Design review of the part built by this model. Coordinates are the model's own, in mm. A direction names the side the tool comes from. Round coordinates to 2 decimals unless told otherwise and drop trailing zeros. Loops run counter-clockwise (first coordinate to the right, second up) from the corner with the lowest first, then second, coordinate; pieces in that order, holes last. Notation, with made-up numbers: (-16.5, 82) - (-5.5, 82) arc R16 cw to (-5.5, 104) - close; hole circle Ø6 at (29, 39). An arc over 180 degrees is marked (long way). Answer as CSV lines item,"result". Start each with the question number.
(1) Consider section D-D (y = 2.5). Give the boundary of the cut face in (x, z).
(2) Consider section A-A (z = 0). Give the boundary of the cut face in (x, y) (3 decimals).
(3) Mouldability with a two-part tool opening along X and no side actions: class faces 1 (the cylindrical face through (7.7, 22.9, 10.1)), 2 (the flat face through (-3, 25.4, -3)), 3 (the flat face through (-1, 3.505, -1)) as released by +X, released by -X, zero draft, split by the parting line, or undercut.
(4) Consider section C-C (z = 9). Give the boundary of the cut face in (x, y), and give its area (3 significant figures).
(5) Consider section B-B (x = 0). Give the boundary of the cut face in (y, z) (3 decimals), and give its area (3 significant figures).
(6) For P1, Ø3, axis at x = -2.5, y = 23, coming from the -Z side; P2, Ø4, axis at y = 9, z = -3, coming from the +X side; P3, Ø4, axis at x = 0, z = 9.525, coming from the -Y side; P4, Ø8, axis at x = 0, z = 0, coming from the +Y side, all flat-tipped, find the tip position at first contact; note any pin that passes through.
(7) For faces 4 (the cylindrical face through (-3.778, 14.84, 0.496)), 5 (the cylindrical face through (3.86, 10.3, 5.04)), 6 (the cylindrical face through (0.773, 22.896, 10.533)), list the 3-axis set-ups (+Z, -Z, +X, -X, +Y, -Y) from which the entire face can be reached by the end or side of a thin tool; tool diameter is ignored.
(8) Wall thickness on L1, parallel to X at y = 23.75, z = 1; L2, parallel to Y at x = -9.75, z = 5.25; L3, parallel to Z at x = 6.5, y = 24.5: over which ranges is each line inside the solid? List them lowest first.
from build123d import *

# Parameters (mm, degrees)
SKETCH2_R          = 2.54
CUT_EXTRUDE1_DEPTH = 3.5052
SKETCH4_R          = 1.27
CUT_EXTRUDE2_DEPTH = 32.108519733
CIRPATTERN1_COUNT  = 8


with BuildPart() as part:
    # Sketch1 → Revolve1 (revolve)
    with BuildSketch(Plane.XY, mode=Mode.PRIVATE) as revolve1_sk:
        Polygon((3.81, 25.4), (3.81, 4.572), (0.635, 4.572), (0.635, 0), (6.35, 0), (6.35, 20.32), (12.7, 20.32), (12.7, 25.4), align=None)
    revolve(revolve1_sk.sketch.rotate(Axis((0, 0, 0), (0, 1, 0)), 90), axis=Axis((0, 0, 0), (0, 1, 0)))

    # Sketch2 → Cut-Extrude1 (cut)
    with BuildSketch(Plane.XZ):
        with Locations(Location((0, 0, 0), (0, 0, 270))):
            Circle(SKETCH2_R)
    extrude(amount=-CUT_EXTRUDE1_DEPTH, mode=Mode.SUBTRACT)

    # Sketch4 → Cut-Extrude2 (cut, through all)
    with BuildSketch(Plane(origin=(0, 25.4, 0), x_dir=(1, 0, 0), z_dir=(0, 1, 0))):
        with Locations(Location((0, 9.525, 0), (0, 0, 270))):
            Circle(SKETCH4_R)
    cut_extrude2 = extrude(amount=-CUT_EXTRUDE2_DEPTH, mode=Mode.SUBTRACT)

    # CirPattern1: Cut-Extrude2 ×8 about axis
    cirpattern1_axis = Axis((0, 0, 0), (0, 1, 0))
    for i in range(1, CIRPATTERN1_COUNT):
        add(cut_extrude2.rotate(cirpattern1_axis, i * 360 / CIRPATTERN1_COUNT), mode=Mode.SUBTRACT)


solid = part.part
Determined:
1,outline,"circle Ø12.7 at (0, 0); hole circle Ø5.08 at (0, 0)"
2,outline,"(-12.7, 20.32) - (-10.795, 20.32) - (-10.795, 25.4) - (-12.7, 25.4) - close; (-8.255, 20.32) - (-6.35, 20.32) - (-6.35, 0) - (-2.54, 0) - (-2.54, 3.505) - (-0.635, 3.505) - (-0.635, 4.572) - (-3.81, 4.572) - (-3.81, 25.4) - (-8.255, 25.4) - close; (0.635, 3.505) - (2.54, 3.505) - (2.54, 0) - (6.35, 0) - (6.35, 20.32) - (8.255, 20.32) - (8.255, 25.4) - (3.81, 25.4) - (3.81, 4.572) - (0.635, 4.572) - close; (10.795, 20.32) - (12.7, 20.32) - (12.7, 25.4) - (10.795, 25.4) - close"
3,face 1,"split by the parting line"
3,face 2,"zero draft"
3,face 3,"undercut"
4,outline,"(-8.96, 20.32) - (-1.16, 20.32) - (-1.16, 25.4) - (-8.96, 25.4) - close; (1.16, 20.32) - (8.96, 20.32) - (8.96, 25.4) - (1.16, 25.4) - close"
4,area,"79.3 mm^2"
5,outline,"(0, -6.35) - (20.32, -6.35) - (20.32, -8.255) - (25.4, -8.255) - (25.4, -3.81) - (4.572, -3.81) - (4.572, -0.635) - (3.505, -0.635) - (3.505, -2.54) - (0, -2.54) - close; (0, 2.54) - (3.505, 2.54) - (3.505, 0.635) - (4.572, 0.635) - (4.572, 3.81) - (25.4, 3.81) - (25.4, 8.255) - (20.32, 8.255) - (20.32, 6.35) - (0, 6.35) - close; (20.32, -12.7) - (25.4, -12.7) - (25.4, -10.795) - (20.32, -10.795) - close; (20.32, 10.795) - (25.4, 10.795) - (25.4, 12.7) - (20.32, 12.7) - close"
5,area,"183 mm^2"
6,P1,"stops at z = -12.66"
6,P2,"stops at x = 6.27"
6,P3,"stops at y = 20.32"
6,P4,"stops at y = 25.4"
7,face 4,"+Y"
7,face 5,"-Y"
7,face 6,"+Y, -Y"
8,L1,"x = -12.66 to -10.31, -8.74 to -3.68, 3.68 to 8.74, 10.31 to 12.66"
8,L2,"y = 20.32 to 25.4"
8,L3,"z = -10.91 to -7.98, -5.49 to 5.49, 7.98 to 10.91"
